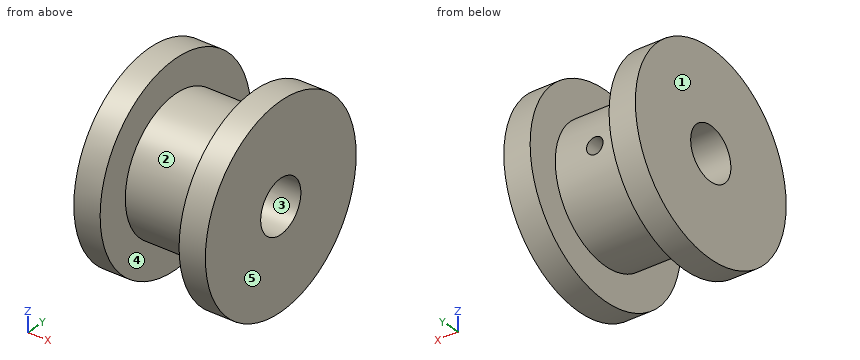
from build123d import *

# Parameters (mm, degrees)
M3_TAPPED_HOLE1_REACH  = 32.822
M3_TAPPED_HOLE1_BORE_R = 1.25


with BuildPart() as part:
    # Sketch1 → Revolve1 (revolve)
    with BuildSketch(Plane(origin=(0, 0, 0), x_dir=(1, 0, 0), z_dir=(0, 1, 0)), mode=Mode.PRIVATE) as revolve1_sk:
        Polygon((0, 4), (20, 4), (20, 15), (16, 15), (16, 10), (4, 10), (4, 15), (0, 15), align=None)
    revolve(revolve1_sk.sketch.rotate(Axis((0, 0, 0), (1, 0, 0)), 180), axis=Axis((0, 0, 0), (1, 0, 0)))

    # M3 Tapped Hole1 bore (on position points) → M3 Tapped Hole1 (cut, up to next)
    with BuildSketch(Plane(origin=(10, 10, 0), x_dir=(0, 0, 1), z_dir=(0, 1, 0)), mode=Mode.PRIVATE) as m3_tapped_hole1_sk1:
        Circle(M3_TAPPED_HOLE1_BORE_R)
    m3_tapped_hole1_tool1 = extrude(m3_tapped_hole1_sk1.sketch, amount=-M3_TAPPED_HOLE1_REACH, mode=Mode.PRIVATE) & part.part
    add(m3_tapped_hole1_tool1.solids().sort_by_distance((10, 10, 0))[0], mode=Mode.SUBTRACT)


solid = part.part
Source: CAD feature listing. Evaluate the final solid. Frame: model axes, mm. Face numbers are marked on the shaded views. A direction names the side the tool comes from. Give positions to 0.01 mm unless a question says otherwise; leave off trailing zeros. Loops run counter-clockwise (first coordinate to the right, second up) from the corner with the lowest first, then second, coordinate; pieces in that order, holes last. Notation, with made-up numbers: (69, 32) -> (118, 32) arc R21 ccw to (118, 54) -> close; hole circle Ø6 at (51.5, -34.75). An arc over 180 degrees is marked (long way). Use a Markdown table: item, result. Add a question column.
1) Section query A-A, the plane y = 0. Return the cut outline in (x, z).
2) Section query C-C, the plane y = 8.25. Return the cut outline in (x, z), then the cut area to 3 significant figures.
3) Section query B-B, the plane z = 0. Return the cut outline in (x, y).
4) Pull-direction query (X, two-part tool) for the marked faces 1, 2 and 3; classes: +X half, -X half, draft (parallel to the pull), parting line (faces both ways), or undercut.
5) Section query D-D, the plane x = 15.25. Return the cut outline in (y, z), then the cut area to 3 significant figures.
6) First-contact query: pin 1 (5 mm diameter, centred on y = 0, z = 0, fed in from -X); pin 2 (10 mm diameter, centred on x = 16.5, z = -0.5, fed in from -Y); pin 3 (5 mm diameter, centred on x = 10, y = -9.5, fed in from -Z); pin 4 (8 mm diameter, centred on x = 10.5, z = -0.5, fed in from -Y). Flat tips, straight axial feed; report the tip coordinate or a pass-through.
7) Line query: line 1 along Y through (x, z) = (7, 0); line 2 along X through (y, z) = (8, 0); line 3 along X through (y, z) = (-10, 7.25). Output: solid intervals per line, ascending. Write a range as [from, to].
8) Reachability of the marked faces 4 and 5 from +Z, -Z, +X, -X, +Y, -Y: full face, straight path, thin tool, end or side. Return the list, or none.
Numbers:
| question | item | result |
|---|---|---|
| 1 | outline | (0, -15) -> (4, -15) -> (4, -10) -> (16, -10) -> (16, -15) -> (20, -15) -> (20, -4) -> (0, -4) -> close; (0, 4) -> (20, 4) -> (20, 15) -> (16, 15) -> (16, 10) -> (4, 10) -> (4, 15) -> (0, 15) -> close |
| 2 | outline | (0, -12.53) -> (4, -12.53) -> (4, -5.65) -> (16, -5.65) -> (16, -12.53) -> (20, -12.53) -> (20, 12.53) -> (16, 12.53) -> (16, 5.65) -> (4, 5.65) -> (4, 12.53) -> (0, 12.53) -> close; hole circle Ø2.5 at (10, 0) |
| 2 | area | 331 mm2 |
| 3 | outline | (0, -15) -> (4, -15) -> (4, -10) -> (16, -10) -> (16, -15) -> (20, -15) -> (20, -4) -> (0, -4) -> close; (0, 4) -> (8.75, 4) -> (8.75, 10) -> (4, 10) -> (4, 15) -> (0, 15) -> close; (11.25, 4) -> (20, 4) -> (20, 15) -> (16, 15) -> (16, 10) -> (11.25, 10) -> close |
| 4 | face 1 | -X half |
| 4 | face 2 | undercut |
| 4 | face 3 | draft |
| 5 | outline | circle Ø20 at (0, 0); hole circle Ø8 at (0, 0) |
| 5 | area | 264 mm2 |
| 6 | pin 1 | passes through |
| 6 | pin 2 | stops at y = -15 |
| 6 | pin 3 | stops at z = -7.14 |
| 6 | pin 4 | stops at y = -10 |
| 7 | line 1 | y = [-10, -4], [4, 10] |
| 7 | line 2 | x = [0, 8.75], [11.25, 20] |
| 7 | line 3 | x = [0, 4], [16, 20] |
| 8 | face 4 | none |
| 8 | face 5 | +Z, -Z, +X, +Y, -Y |
